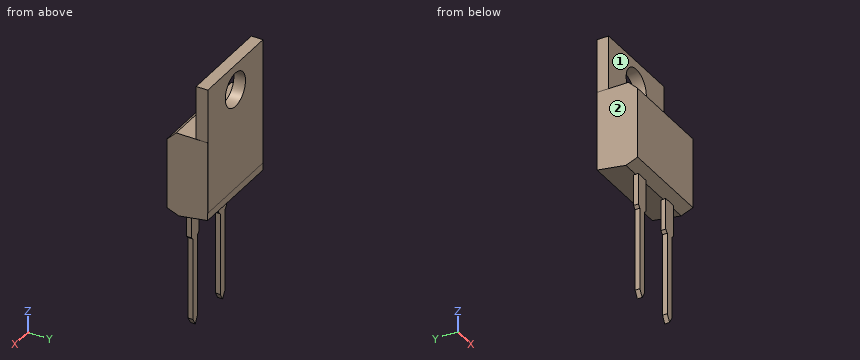
from build123d import *

# Parameters (mm, degrees)
SKETCH004_W  = 10.23
SKETCH004_H  = 1.27
PAD002_DEPTH = 13.775
SKETCH005_R  = 1.8675
POCKET_DEPTH = 1.271
PAD_DEPTH    = 0.2625
PAD001_DEPTH = 5.125


with BuildPart() as pocket:
    # Sketch004 → Pad002 (new body)
    with BuildSketch(Plane.XY.offset(5)):
        with Locations((2.54, 2.525)):
            Rectangle(SKETCH004_W, SKETCH004_H)
    extrude(amount=PAD002_DEPTH)

    # Sketch005 → Pocket (cut, through all)
    with BuildSketch(Plane(origin=(0, 1.89, 5), x_dir=(1, 0, 0), z_dir=(0, -1, 0))):
        with Locations((2.54, 11.005)):
            Circle(SKETCH005_R)
    extrude(amount=-POCKET_DEPTH, mode=Mode.SUBTRACT)


with BuildPart() as pad:
    # Sketch → Pad (new body, symmetric)
    with BuildSketch(Plane.XZ):
        Polygon((-0.73, 0.3025), (-0.4275, 0), (-0.4275, -9.009548), (0, -9.75), (0.4275, -9.009548), (0.4275, 0), (0.73, 0.3025), (0.73, 3.73), (-0.73, 3.73), align=None)
        Polygon((4.35, 0.3025), (4.6525, 0), (4.6525, -9.009548), (5.08, -9.75), (5.5075, -9.009548), (5.5075, 0), (5.81, 0.3025), (5.81, 3.73), (4.35, 3.73), align=None)
    extrude(amount=PAD_DEPTH, both=True)


with BuildPart() as to_220_2_vertical:
    # Sketch001 → Pad001 (new body, symmetric)
    with BuildSketch(Plane.YZ.offset(2.54)):
        Polygon((0, 3.685), (-1.295, 4.185), (-1.295, 11.875), (-0.295, 12.875), (3.15, 12.875), (3.15, 4.185), align=None)
    extrude(amount=PAD001_DEPTH, both=True)

    add(pocket.part)
    add(pad.part)


solid = to_220_2_vertical.part
Work out the finished part from the listing and answer in its coordinate system (mm). Face numbers are marked on the shaded views. A direction names the side the tool comes from. Round coordinates to 2 decimals unless told otherwise and drop trailing zeros. Write each loop counter-clockwise with the first axis right and the second up, starting at its lowest first coordinate (ties: lowest second). Pieces come first, ordered by that corner, then holes. Notation, with made-up numbers: (84.5, 82.5) -> (108.5, 82.5) arc R33 cw to (108.5, 116.5) -> close; hole circle Ø9 at (-9.5, 46). An arc over 180 degrees is marked (long way). Answer as CSV lines item,"result". Start each with the question number.
(1) The part is cut by section A-A, the plane z = -0.25. Give the vertices of the cut face in (x, y), then the cut area to 3 significant figures.
(2) The part is cut by section D-D, the plane x = 6.5. Give the vertices of the cut face in (y, z) (3 decimals).
(3) Each of these flat-tipped pins is pushed along its axis until it touches: pin 1 (0.6 mm diameter, centred on y = 0, z = -5.5, fed in from -X); pin 2 (1 mm diameter, centred on x = 0.5, y = 2.5, fed in from -Z); pin 3 (0.7 mm diameter, centred on x = -0.5, z = -3.5, fed in from +Y). Where does it stop, or does it pass through?
(4) Find the intervals of material crossed by probe 1 along Z at (x, y) = (2.54, 2.2) (1 decimal); probe 2 along Z at (x, y) = (2.54, 2.8) (1 decimal); probe 3 along Z at (x, y) = (1.75, -0.85), in increasing order.
(5) A tool of negligible diameter and unlimited length cuts with its end or side. For the marked faces 1 and 2, from which of +Z, -Z, +X, -X, +Y, -Y can it reach the whole face along a straight path? Write none if from no direction.
Output values:
1,outline,"(-0.43, -0.26) -> (0.43, -0.26) -> (0.43, 0.26) -> (-0.43, 0.26) -> close; (4.65, -0.26) -> (5.51, -0.26) -> (5.51, 0.26) -> (4.65, 0.26) -> close"
1,area,"0.898 mm²"
2,outline,"(-1.295, 4.185) -> (0, 3.685) -> (3.15, 4.185) -> (3.15, 5) -> (3.16, 5) -> (3.16, 18.775) -> (1.89, 18.775) -> (1.89, 12.875) -> (-0.295, 12.875) -> (-1.295, 11.875) -> close"
3,pin 1,"stops at x = -0.43"
3,pin 2,"stops at z = 4"
3,pin 3,"stops at y = 0.26"
4,probe 1,"z = 4 to 14.1, 17.9 to 18.8"
4,probe 2,"z = 4.1 to 14.1, 17.9 to 18.8"
4,probe 3,"z = 4.01 to 12.32"
5,face 1,"+Z, +X, -X, -Y"
5,face 2,"+Z, -Z, -X, +Y, -Y"
